Input: part model. Units: mm. Frame: model coordinates. Face numbers are marked on the shaded views. A direction names the side the tool comes from. Round coordinates to 2 decimals unless told otherwise and drop trailing zeros. Loops run counter-clockwise (first coordinate to the right, second up) from the corner with the lowest first, then second, coordinate; pieces in that order, holes last. Notation, with made-up numbers: (-15, 8.25) -> (10, 8.25) arc R6 ccw to (10, 13.25) -> close; hole circle Ø7 at (64, -3). An arc over 180 degrees is marked (long way). Answer as a JSON object with one key per item and string values.
```python
from build123d import *

# Parameters (mm, degrees)
SKETCH_1_W                = 400
SKETCH_1_H                = 320
EXTRUDE_7_DEPTH           = 120
SKETCH_6_R                = 7.620000001
SKETCH_6_R_2              = 7.62
CUT_EXTRUDE_3_DEPTH       = 283.842712475
CUT_EXTRUDE_START         = -120
SKETCH_7_W                = 185
SKETCH_7_H                = 320
CUT_EXTRUDE_4_DEPTH       = 114
SKETCH_8_W                = 310
SKETCH_8_H                = 94
CUT_EXTRUDE_5_DEPTH       = 448.2135955
SKETCH_10_R               = 10
CUT_EXTRUDE_7_DEPTH       = 396.979797464
CUT_EXTRUDE_8_REACH       = 284.843
SKETCH_12_R               = 10
SKETCH_13_R               = 2
CUT_EXTRUDE_9_DEPTH       = 20
CUT_EXTRUDE_12_DEPTH      = 281.349781523
CUT_EXTRUDE_12_DEPTH_BACK = 281.349781523
SKETCH_14_W               = 100
SKETCH_14_H               = 100
CUT_EXTRUDE_13_REACH      = 284.843
SKETCH_15_W               = 165
SKETCH_15_H               = 140


with BuildPart() as part:
    # 草图1 → 凸台-拉伸7 (new body)
    with BuildSketch(Plane(origin=(0, 0, 0), x_dir=(1, 0, 0), z_dir=(0, 1, 0))):
        Rectangle(SKETCH_1_W, SKETCH_1_H)
    extrude(amount=EXTRUDE_7_DEPTH)

    # 草图6 → 切除-拉伸3 (cut, through all)
    with BuildSketch(Plane(origin=(0, 120, 0), x_dir=(1, 0, 0), z_dir=(0, 1, 0))):
        with Locations(Location((-180, -71.4375, 0), (0, 0, 270))):
            Circle(SKETCH_6_R)
        with Locations(Location((-165.712492884, 57.173286175, 0), (0, 0, 270))):
            Circle(SKETCH_6_R_2)
        with Locations(Location((-165.7125, -57.126713825, 0), (0, 0, 270))):
            Circle(SKETCH_6_R_2)
        with Locations(Location((-180, 71.4375, 0), (0, 0, 270))):
            Circle(SKETCH_6_R_2)
        with Locations(Location((-37.125, 71.4375, 0), (0, 0, 270))):
            Circle(SKETCH_6_R_2)
        with Locations(Location((-51.412502372, 57.126713825, 0), (0, 0, 270))):
            Circle(SKETCH_6_R_2)
        with Locations(Location((-51.412509488, -57.173286175, 0), (0, 0, 270))):
            Circle(SKETCH_6_R_2)
        with Locations(Location((-37.125, -71.4375, 0), (0, 0, 270))):
            Circle(SKETCH_6_R_2)
    extrude(amount=-CUT_EXTRUDE_3_DEPTH, mode=Mode.SUBTRACT)

    # 草图7 → 切除-拉伸4 (cut)
    with BuildSketch(Plane(origin=(0, 120, 0), x_dir=(1, 0, 0), z_dir=(0, 1, 0)).offset(CUT_EXTRUDE_START)):
        with Locations((-107.5, 0)):
            Rectangle(SKETCH_7_W, SKETCH_7_H)
    extrude(amount=CUT_EXTRUDE_4_DEPTH, mode=Mode.SUBTRACT)

    # 草图8 → 切除-拉伸5 (cut, through all)
    with BuildSketch(Plane(origin=(200, 0, 0), x_dir=(0, 0, -1), z_dir=(1, 0, 0))):
        with Locations((0, 53)):
            Rectangle(SKETCH_8_W, SKETCH_8_H)
    extrude(amount=-CUT_EXTRUDE_5_DEPTH, mode=Mode.SUBTRACT)

    # 草图10 → 切除-拉伸7 (cut, through all)
    with BuildSketch(Plane.XY.offset(160)):
        with Locations((90, 60)):
            Circle(SKETCH_10_R)
    extrude(amount=-CUT_EXTRUDE_7_DEPTH, mode=Mode.SUBTRACT)

    # 草图12 → 切除-拉伸8 (cut, up to next)
    with BuildSketch(Plane(origin=(0, 120, 0), x_dir=(1, 0, 0), z_dir=(0, 1, 0)), mode=Mode.PRIVATE) as cut_extrude_8_sk1:
        with Locations(Location((5, 90, 0), (0, 0, 270))):
            Circle(SKETCH_12_R)
    cut_extrude_8_tool1 = extrude(cut_extrude_8_sk1.sketch, amount=-CUT_EXTRUDE_8_REACH, mode=Mode.PRIVATE) & part.part
    # 草图12 → 切除-拉伸8 (cut, up to next)
    with BuildSketch(Plane(origin=(0, 120, 0), x_dir=(1, 0, 0), z_dir=(0, 1, 0)), mode=Mode.PRIVATE) as cut_extrude_8_sk2:
        with Locations(Location((5, 0, 0), (0, 0, 270))):
            Circle(SKETCH_12_R)
    cut_extrude_8_tool2 = extrude(cut_extrude_8_sk2.sketch, amount=-CUT_EXTRUDE_8_REACH, mode=Mode.PRIVATE) & part.part
    # 草图12 → 切除-拉伸8 (cut, up to next)
    with BuildSketch(Plane(origin=(0, 120, 0), x_dir=(1, 0, 0), z_dir=(0, 1, 0)), mode=Mode.PRIVATE) as cut_extrude_8_sk3:
        with Locations(Location((5, 30, 0), (0, 0, 270))):
            Circle(SKETCH_12_R)
    cut_extrude_8_tool3 = extrude(cut_extrude_8_sk3.sketch, amount=-CUT_EXTRUDE_8_REACH, mode=Mode.PRIVATE) & part.part
    # 草图12 → 切除-拉伸8 (cut, up to next)
    with BuildSketch(Plane(origin=(0, 120, 0), x_dir=(1, 0, 0), z_dir=(0, 1, 0)), mode=Mode.PRIVATE) as cut_extrude_8_sk4:
        with Locations(Location((5, 60, 0), (0, 0, 270))):
            Circle(SKETCH_12_R)
    cut_extrude_8_tool4 = extrude(cut_extrude_8_sk4.sketch, amount=-CUT_EXTRUDE_8_REACH, mode=Mode.PRIVATE) & part.part
    # 草图12 → 切除-拉伸8 (cut, up to next)
    with BuildSketch(Plane(origin=(0, 120, 0), x_dir=(1, 0, 0), z_dir=(0, 1, 0)), mode=Mode.PRIVATE) as cut_extrude_8_sk5:
        with Locations(Location((5, -30, 0), (0, 0, 270))):
            Circle(SKETCH_12_R)
    cut_extrude_8_tool5 = extrude(cut_extrude_8_sk5.sketch, amount=-CUT_EXTRUDE_8_REACH, mode=Mode.PRIVATE) & part.part
    # 草图12 → 切除-拉伸8 (cut, up to next)
    with BuildSketch(Plane(origin=(0, 120, 0), x_dir=(1, 0, 0), z_dir=(0, 1, 0)), mode=Mode.PRIVATE) as cut_extrude_8_sk6:
        with Locations(Location((5, -60, 0), (0, 0, 270))):
            Circle(SKETCH_12_R)
    cut_extrude_8_tool6 = extrude(cut_extrude_8_sk6.sketch, amount=-CUT_EXTRUDE_8_REACH, mode=Mode.PRIVATE) & part.part
    # 草图12 → 切除-拉伸8 (cut, up to next)
    with BuildSketch(Plane(origin=(0, 120, 0), x_dir=(1, 0, 0), z_dir=(0, 1, 0)), mode=Mode.PRIVATE) as cut_extrude_8_sk7:
        with Locations(Location((5, -90, 0), (0, 0, 270))):
            Circle(SKETCH_12_R)
    cut_extrude_8_tool7 = extrude(cut_extrude_8_sk7.sketch, amount=-CUT_EXTRUDE_8_REACH, mode=Mode.PRIVATE) & part.part
    # 草图12 → 切除-拉伸8 (cut, up to next)
    with BuildSketch(Plane(origin=(0, 120, 0), x_dir=(1, 0, 0), z_dir=(0, 1, 0)), mode=Mode.PRIVATE) as cut_extrude_8_sk8:
        with Locations(Location((5, 120, 0), (0, 0, 270))):
            Circle(SKETCH_12_R)
    cut_extrude_8_tool8 = extrude(cut_extrude_8_sk8.sketch, amount=-CUT_EXTRUDE_8_REACH, mode=Mode.PRIVATE) & part.part
    # 草图12 → 切除-拉伸8 (cut, up to next)
    with BuildSketch(Plane(origin=(0, 120, 0), x_dir=(1, 0, 0), z_dir=(0, 1, 0)), mode=Mode.PRIVATE) as cut_extrude_8_sk9:
        with Locations(Location((5, -120, 0), (0, 0, 270))):
            Circle(SKETCH_12_R)
    cut_extrude_8_tool9 = extrude(cut_extrude_8_sk9.sketch, amount=-CUT_EXTRUDE_8_REACH, mode=Mode.PRIVATE) & part.part
    add(cut_extrude_8_tool1.solids().sort_by_distance((5, 120, -90))[0], mode=Mode.SUBTRACT)
    add(cut_extrude_8_tool2.solids().sort_by_distance((5, 120, 0))[0], mode=Mode.SUBTRACT)
    add(cut_extrude_8_tool3.solids().sort_by_distance((5, 120, -30))[0], mode=Mode.SUBTRACT)
    add(cut_extrude_8_tool4.solids().sort_by_distance((5, 120, -60))[0], mode=Mode.SUBTRACT)
    add(cut_extrude_8_tool5.solids().sort_by_distance((5, 120, 30))[0], mode=Mode.SUBTRACT)
    add(cut_extrude_8_tool6.solids().sort_by_distance((5, 120, 60))[0], mode=Mode.SUBTRACT)
    add(cut_extrude_8_tool7.solids().sort_by_distance((5, 120, 90))[0], mode=Mode.SUBTRACT)
    add(cut_extrude_8_tool8.solids().sort_by_distance((5, 120, -120))[0], mode=Mode.SUBTRACT)
    add(cut_extrude_8_tool9.solids().sort_by_distance((5, 120, 120))[0], mode=Mode.SUBTRACT)

    # 草图13 → 切除-拉伸9 (cut)
    with BuildSketch(Plane(origin=(200, 0, 0), x_dir=(0, 0, -1), z_dir=(1, 0, 0))):
        with Locations((0, 3)):
            Circle(SKETCH_13_R)
        with Locations((19, 3)):
            Circle(SKETCH_13_R)
        with Locations((38, 3)):
            Circle(SKETCH_13_R)
        with Locations((57, 3)):
            Circle(SKETCH_13_R)
        with Locations((-57, 3)):
            Circle(SKETCH_13_R)
        with Locations((-38, 3)):
            Circle(SKETCH_13_R)
        with Locations((-19, 3)):
            Circle(SKETCH_13_R)
    extrude(amount=-CUT_EXTRUDE_9_DEPTH, mode=Mode.SUBTRACT)

    # 草图14 → 切除-拉伸12 (cut, two sides: drawn at the far end of the back side and taken through both)
    with BuildSketch(Plane(origin=(0, 6, 0), x_dir=(1, 0, 0), z_dir=(0, 1, 0)).offset(-CUT_EXTRUDE_12_DEPTH_BACK)):
        with Locations((110, 0)):
            Rectangle(SKETCH_14_W, SKETCH_14_H)
    extrude(amount=CUT_EXTRUDE_12_DEPTH + CUT_EXTRUDE_12_DEPTH_BACK, mode=Mode.SUBTRACT)

    # 草图15 → 切除-拉伸13 (cut, up to next)
    with BuildSketch(Plane(origin=(0, 120, 0), x_dir=(1, 0, 0), z_dir=(0, 1, 0)), mode=Mode.PRIVATE) as cut_extrude_13_sk1:
        with Locations((117.5, 0)):
            Rectangle(SKETCH_15_W, SKETCH_15_H)
    cut_extrude_13_tool1 = extrude(cut_extrude_13_sk1.sketch, amount=-CUT_EXTRUDE_13_REACH, mode=Mode.PRIVATE) & part.part
    add(cut_extrude_13_tool1.solids().sort_by_distance((117.5, 120, 0))[0], mode=Mode.SUBTRACT)


solid = part.part
```
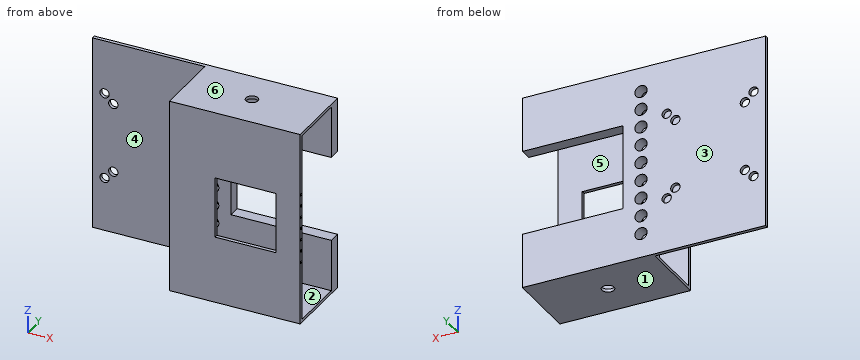
1) Reachability of the marked faces 4, 5 and 6 from +Z, -Z, +X, -X, +Y, -Y: full face, straight path, thin tool, end or side. Return the list, or none.
Output:
{"face 4": "+Z, -Z, -X, -Y", "face 5": "+X, -X", "face 6": "+Z, +X, -X, +Y, -Y"}
2) Ray query, probe 1 along X at (y, z) = (102.5, -121); probe 2 along Z at (x, y) = (73.5, 39); probe 3 along Y at (x, z) = (101.5, 109). Return the intervals inside material, ascending.
Output:
{"probe 1": "x = -15 to -4.95, 14.95 to 200", "probe 2": "z = -160 to -155, 155 to 160", "probe 3": "y = 0 to 6, 100 to 120"}
3) Section D-D, the plane y = 60. Output: boundary loops of the cut face in (x, z), plus the area to 3 significant figures.
Output:
{"outline": "(-15, -160) -> (80, -160) -> (80, -155) -> (-15, -155) -> close; (-15, 155) -> (80, 155) -> (80, 160) -> (-15, 160) -> close; (100, -160) -> (200, -160) -> (200, -155) -> (100, -155) -> close; (100, 155) -> (200, 155) -> (200, 160) -> (100, 160) -> close", "area": "1,950 mm^2"}
4) Draft query along Z for the marked faces 1, 2 and 3. Return one class per face: +Z half, -Z half, draft (parallel to the pull), parting line (faces both ways), or undercut.
Output:
{"face 1": "-Z half", "face 2": "undercut", "face 3": "draft"}
5) Section C-C, the plane x = 151.5. Output: boundary loops of the cut face in (y, z), plus the area to 3 significant figures.
Output:
{"outline": "(0, -160) -> (120, -160) -> (120, -70) -> (100, -70) -> (100, -155) -> (6, -155) -> (6, -50) -> (0, -50) -> close; (0, 50) -> (6, 50) -> (6, 155) -> (100, 155) -> (100, 70) -> (120, 70) -> (120, 160) -> (0, 160) -> close", "area": "5,860 mm^2"}
6) Section B-B, the plane z = -90. Output: boundary loops of the cut face in (x, y).
Output:
{"outline": "(-200, 114) -> (-15, 114) -> (-15, 100) -> (-5, 100) -> (-5, 120) -> (-200, 120) -> close; (-15, 0) -> (200, 0) -> (200, 6) -> (-15, 6) -> close; (15, 100) -> (200, 100) -> (200, 120) -> (15, 120) -> close"}
7) Contact query for flat-ended pins moving along their axis: P1, Ø24.5, axis at x = -37.12, z = -71.44, coming from the -Y side; P2, Ø3, axis at y = 3, z = -19, coming from the +X side; P3, Ø9, axis at x = -165.71, z = 57.13, coming from the -Y side; P4, Ø18, axis at x = 5, z = 120, coming from the +Y side. Output: stop coordinate, or through.
Output:
{"P1": "stops at y = 114", "P2": "stops at x = 180", "P3": "passes through", "P4": "stops at y = 6"}
8) Section A-A, the plane y = 19. Output: boundary loops of the cut face in (x, z).
Output:
{"outline": "(-15, -160) -> (200, -160) -> (200, -155) -> (-15, -155) -> close; (-15, 155) -> (200, 155) -> (200, 160) -> (-15, 160) -> close"}
